Job drawing, mm, ordinate dimensions from the low corner. One solid piece. Round coordinates to 2 decimals unless told otherwise and drop trailing zeros. Loops run counter-clockwise (first coordinate to the right, second up) from the corner with the lowest first, then second, coordinate; pieces in that order, holes last.
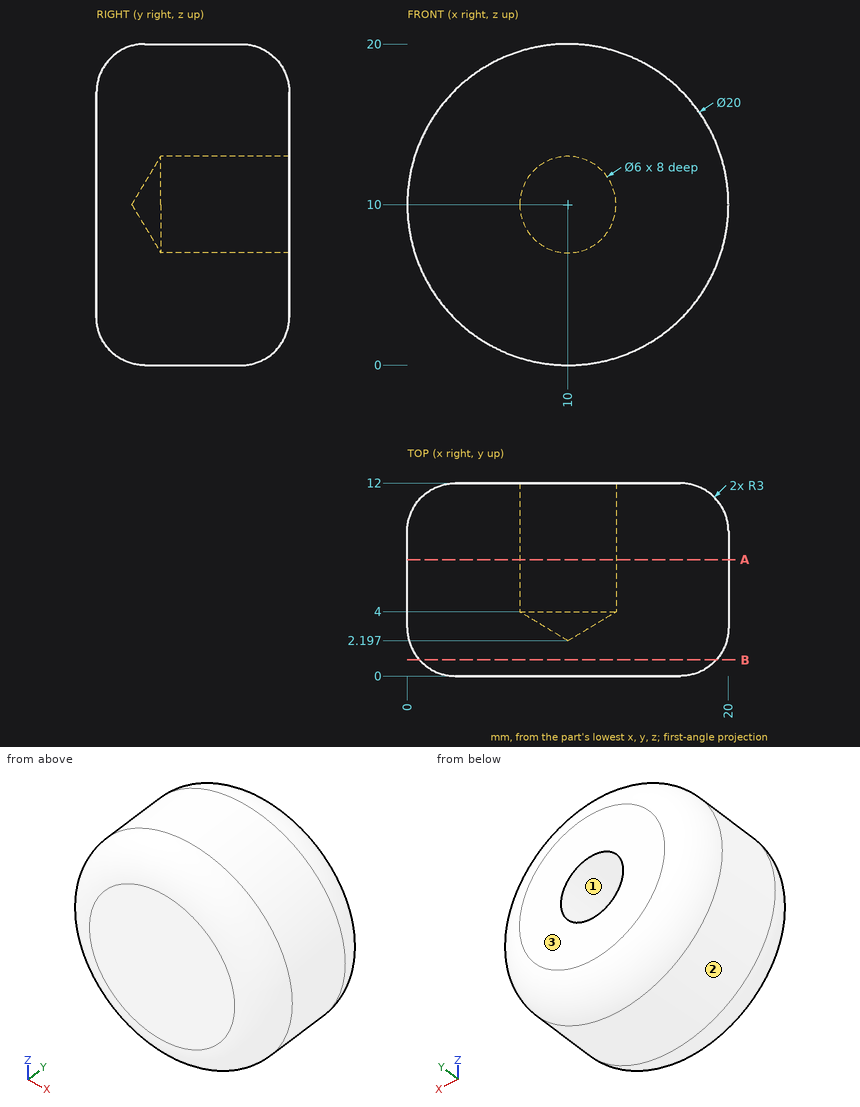
Item 1: Probe line 1 (Z direction, x = 10, y = 6); line 2 (X direction, y = 4.25, z = 10.5); line 3 (Y direction, x = 5, z = 15.25). List the from-to ranges inside material, lowest first.
Answers follow:
line 1: z = 0 to 7, 13 to 20
line 2: x = 0.01 to 7.04, 12.96 to 19.99
line 3: y = 0.01 to 11.99
Item 2: Two-plate mould, pull along Z, no slides. Class the marked faces 1, 2 and 3: released by +Z, released by -Z, zero draft, split by the parting line, or undercut.
Answers follow:
face 1: undercut
face 2: split by the parting line
face 3: zero draft
Item 3: Flat gauge pins, fed straight in: P1, Ø1.5, axis at y = 2.5, z = 7, coming from the +X side; P2, Ø2, axis at x = 15.5, z = 3.5, coming from the -Y side (1 decimal); P3, Ø3, axis at x = 4.5, z = 17, coming from the +Y side. Where does each tip first touch, or does it go through?
Answers follow:
P1: stops at x = 19.72
P2: stops at y = 0
P3: stops at y = 11.97
Item 4: Cut at B-B, the plane y = 1. Give the cut face in (x, z), plus the area to 3 significant figures.
Answers follow:
outline: circle Ø18.47 at (10, 10)
area: 268 mm2
Item 5: Cut at A-A, the plane y = 7.25. Give the cut face in (x, z).
Answers follow:
outline: circle Ø20 at (10, 10); hole circle Ø6 at (10, 10)
